```python
from build123d import *

# Parameters (mm, degrees)
ESQUISSE1_W                = 43
ESQUISSE1_H                = 23
BOSS_EXTRU_1_DEPTH         = 3
ESQUISSE2_W                = 3
ESQUISSE2_H                = 10
ENL_V_MAT_EXTRU_1_DEPTH    = 3
ESQUISSE3_W                = 10
ESQUISSE3_H                = 3
ENL_V_MAT_EXTRU_2_DEPTH    = 3
R_P_TITION_LIN_AIRE1_COUNT = 2
R_P_TITION_LIN_AIRE1_PITCH = 20


with BuildPart() as part:
    # Esquisse1 → Boss.-Extru.1 (new body)
    with BuildSketch(Plane.XY):
        with Locations((21.5, -11.5)):
            Rectangle(ESQUISSE1_W, ESQUISSE1_H)
    extrude(amount=BOSS_EXTRU_1_DEPTH)

    # Esquisse2 → Enlèv. mat.-Extru.1 (cut)
    with BuildSketch(Plane(origin=(43, 0, 0), x_dir=(0, 0, -1), z_dir=(1, 0, 0))):
        with Locations((-1.5, -18)):
            Rectangle(ESQUISSE2_W, ESQUISSE2_H)
    extrude(amount=-ENL_V_MAT_EXTRU_1_DEPTH, mode=Mode.SUBTRACT)

    # Esquisse3 → Enlèv. mat.-Extru.2 (cut)
    with BuildSketch(Plane.XY.offset(3)):
        with Locations((5, -21.5)):
            Rectangle(ESQUISSE3_W, ESQUISSE3_H)
    enl_v_mat_extru_2 = extrude(amount=-ENL_V_MAT_EXTRU_2_DEPTH, mode=Mode.SUBTRACT)

    # Répétition linéaire1: Enlèv. mat.-Extru.2 ×2
    with Locations(*[(i * R_P_TITION_LIN_AIRE1_PITCH, 0, 0) for i in range(1, R_P_TITION_LIN_AIRE1_COUNT)]):
        add(enl_v_mat_extru_2, mode=Mode.SUBTRACT)


solid = part.part
```
Source: CAD feature listing. Evaluate the final solid. Frame: model axes, mm. A direction names the side the tool comes from. Coordinates: 2 decimals unless noted, no trailing zeros. Loops run counter-clockwise (first coordinate to the right, second up) from the corner with the lowest first, then second, coordinate; pieces in that order, holes last. Notation, with made-up numbers: M -15.75,-5 L 41.25,-5 A16 cw 41.25,25 Z; hole C 74.25,72.5 d9. An arc over 180 degrees is marked long. Put each result on its own line as item: value. Start each with the question number.
1) Cut plane B-B on y = -15.25. Return the cut outline in (x, z).
2) Cut plane C-C on x = 25. Return the cut outline in (y, z), then the cut area to 3 significant figures.
3) Contact query for flat-ended pins moving along their axis: pin 1 Ø10 at (x, y) = (5.5, -18.5) entering from -Z; pin 2 Ø0.9 at (x, z) = (2.5, 1.5) entering from -Y; pin 3 Ø1.5 at (y, z) = (-15.5, 1) entering from +X; pin 4 Ø1.5 at (y, z) = (-22, 1) entering from -X. Output: stop coordinate, or through.
4) Pull-direction query (X, two-part tool) for faces 4 (the face through (43, -7, 1)), 5 (the face through (25, -20, 2)), 6 (the face through (35, -23, 1)), 7 (the face through (10, -22, 2)); classes: pulls with the +X half, pulls with the -X half, needs draft (parallel to the pull), parting line crosses it, or undercut.
5) Reachability of faces 1 (the face through (42, -13, 2)), 2 (the face through (5, -20, 2)), 3 (the face through (20, -22, 2)) from +Z, -Z, +X, -X, +Y, -Y: full face, straight path, thin tool, end or side. Return the list, or none.
6) Ray query, L1, parallel to X at y = -21.25, z = 1.2; L2, parallel to X at y = -16.5, z = 1.2; L3, parallel to Y at x = 6.5, z = 0.9. Return the intervals inside material, ascending. Write a range as from..to.
7) Cut plane A-A on z = 1.55. Return the cut outline in (x, y).
The answers:
1. outline: M 0,0 L 40,0 L 40,3 L 0,3 Z
2. outline: M -20,0 L 0,0 L 0,3 L -20,3 Z
2. area: 60.0 mm²
3. pin 1: stops at z = 0
3. pin 2: stops at y = -20
3. pin 3: stops at x = 40
3. pin 4: stops at x = 10
4. face 4: pulls with the +X half
4. face 5: undercut
4. face 6: needs draft
4. face 7: pulls with the -X half
5. face 1: +Z, -Z, +X, -Y
5. face 2: +Z, -Z, -X, -Y
5. face 3: +Z, -Z, -Y
6. L1: x = 10..20, 30..40
6. L2: x = 0..40
6. L3: y = -20..0
7. outline: M 0,-20 L 10,-20 L 10,-23 L 20,-23 L 20,-20 L 30,-20 L 30,-23 L 40,-23 L 40,-13 L 43,-13 L 43,0 L 0,0 Z
